Autodesk Inventor part; units mm, degrees
ref_plane "YZ Plane" through (0, 0, 0) normal (1, 0, 0) x (0, 1, 0)
ref_plane "XZ Plane" through (0, 0, 0) normal (0, 1, 0) x (-1, 0, 0)
ref_plane "XY Plane" through (0, 0, 0) normal (0, 0, 1) x (1, 0, 0)
sketch "Sketch1" plane through (0, 0, 0) normal (0, 1, 0) x (-1, 0, 0)
  line L0 (56, 0) -> (-56, 0)
  line L1 (0, -156) -> (0, 26)
  line L2 (40, 0) -> (-40, 0)
  line L3 (-40, 0) -> (-40, -130)
  line L4 (-40, -130) -> (40, -130)
  line L5 (40, -130) -> (40, 0)
  point P0 (0, 0)
  point P1 (0, 0)
  dimension "d0" = 80
  dimension "d1" = 130
  dimension "d2" = 40
extrude "Extrusion1" add sketch "Sketch1" along normal blind 60
sketch "Sketch2" plane through (0, 60, 0) normal (0, 1, 0) x (1, 0, 0)
  line L0 (-35, 5) -> (35, 5)
  line L1 (35, 5) -> (35, 125)
  line L2 (35, 125) -> (-35, 125)
  line L3 (-35, 125) -> (-35, 5)
  line L4 (-40, 130) -> (-40, 0)
  line L5 (-40, 0) -> (40, 0)
  point P0 (0, 0)
  dimension "d5" = 70
  dimension "d6" = 120
  dimension "d7" = 5
  dimension "d8" = 5
extrude "Extrusion2" cut sketch "Sketch2" against normal blind 50
sketch "Sketch3" plane through (40, 0, 0) normal (1, 0, 0) x (0, 0, -1)
  line L0 (113, 48) -> (123, 48)
  line L1 (123, 48) -> (123, 30)
  line L2 (123, 30) -> (113, 30)
  line L3 (113, 30) -> (113, 48)
  line L4 (130, 0) -> (130, 60)
  line L5 (0, 60) -> (130, 60)
  line L6 (98, 48) -> (108, 48)
  line L7 (108, 48) -> (108, 30)
  line L8 (108, 30) -> (98, 30)
  line L9 (98, 30) -> (98, 48)
  point P0 (0, 0)
  dimension "d11" = 10
  dimension "d12" = 18
  dimension "d13" = 7
  dimension "d14" = 12
  dimension "d15" = 10
  dimension "d16" = 18
  dimension "d17" = 5
extrude "Extrusion3" cut sketch "Sketch3" against normal blind 5
sketch "Sketch4" plane through (40, 0, 0) normal (1, 0, 0) x (0, 0, -1)
  circle A0 centre (115, 15) radius 5
  line L0 (0, 0) -> (130, 0)
  line L1 (130, 0) -> (130, 60)
  dimension "d20" = 10
  dimension "d21" = 15
  dimension "d22" = 15
extrude "Extrusion4" cut sketch "Sketch4" against normal blind 5
sketch "Sketch6" plane through (0, 10, 0) normal (0, 1, 0) x (1, 0, 0)
  line L0 (-35, 125) -> (35, 125)
  line L1 (-35, 5) -> (-35, 125)
  line L2 (35, 5) -> (-35, 5)
  line L3 (35, 115) -> (35, 5)
  line L4 (35, 125) -> (35, 115)
  line L5 (-35, 88) -> (30, 88)
  line L6 (30, 88) -> (30, 78)
  line L7 (30, 78) -> (-35, 78)
  line L8 (-35, 78) -> (-35, 88)
  line L9 (25, 125) -> (25, 88)
  line L10 (25, 88) -> (30, 88)
  line L11 (30, 88) -> (30, 125)
  point P0 (0, 0)
  dimension "d30" = 65
  dimension "d31" = 10
extrude "Extrusion6" add sketch "Sketch6" along normal blind 25 contours L5 L6 L7 L1
sketch "Sketch7" plane through (0, 10, 0) normal (0, 1, 0) x (1, 0, 0)
  line L0 (30, 78) -> (-35, 78)
  line L1 (-35, 5) -> (-35, 78)
  line L2 (35, 5) -> (-35, 5)
  line L3 (35, 115) -> (35, 5)
  line L4 (35, 125) -> (35, 115)
  line L5 (-35, 125) -> (35, 125)
  line L6 (30, 88) -> (30, 78)
  line L7 (-35, 57) -> (30, 57)
  line L8 (30, 57) -> (30, 47)
  line L9 (30, 47) -> (-35, 47)
  line L10 (-35, 47) -> (-35, 57)
  line L11 (30, 88) -> (30, 125)
  line L12 (-35, 88) -> (30, 88)
  line L13 (-35, 88) -> (-35, 125)
  point P0 (0, 0)
  dimension "d34" = 65
  dimension "d35" = 10
  dimension "d36" = 21
extrude "Extrusion7" add sketch "Sketch7" along normal blind 25 contours L7 L8 L9 L1
sketch "Sketch8" plane through (0, 10, 0) normal (0, 1, 0) x (1, 0, 0)
  line L0 (-35, 57) -> (30, 57)
  line L1 (30, 57) -> (30, 47)
  line L2 (30, 47) -> (-35, 47)
  line L3 (-35, 5) -> (-35, 47)
  line L4 (35, 5) -> (-35, 5)
  line L5 (35, 115) -> (35, 5)
  line L6 (35, 125) -> (35, 115)
  line L7 (-35, 125) -> (35, 125)
  line L8 (30, 88) -> (30, 78)
  line L9 (30, 78) -> (-35, 78)
  line L10 (-35, 57) -> (-35, 78)
  line L11 (-35, 78) -> (-25, 78)
  line L12 (-25, 78) -> (-25, 57)
  line L13 (-25, 57) -> (-35, 57)
  line L14 (-35, 57) -> (-35, 78)
  line L15 (16, 58) -> (16, 79)
  line L16 (16, 79) -> (26, 79)
  line L17 (26, 79) -> (26, 57)
  line L18 (26, 57) -> (16, 57)
  line L19 (16, 57) -> (16, 79)
  line L20 (30, 57) -> (-35, 57)
  line L21 (-35, 88) -> (-35, 125)
  line L22 (-35, 88) -> (30, 88)
  point P0 (0, 0)
  dimension "d39" = 10
  dimension "d40" = 10
  dimension "d41" = 41
extrude "Extrusion8" add sketch "Sketch8" along normal blind 20 contours L10 L9 L12 L0 | L19 L15 L9 L17 L0 | L15 L16 L17 L9
sketch "Sketch10" plane through (-40, 0, 0) normal (0, 0, 1) x (1, 0, 0)
  circle A0 centre (22, 40) radius 1.625
  circle A1 centre (40, 40) radius 1.625
  circle A2 centre (58, 40) radius 1.625
  line L0 (0, 0) -> (0, 60)
  line L1 (0, 0) -> (80, 0)
  line L2 (80, 0) -> (80, 60)
  line L3 (0, 60) -> (80, 60)
  line L4 (0, 0) -> (0, 60)
  point P0 (40, 0)
  dimension "d49" = 3.25
  dimension "d51" = 3.25
  dimension "d53" = 3.25
  dimension "d55" = 18
  dimension "d56" = 18
  dimension "d59" = 22
  dimension "d60" = 22
  dimension "d61" = 20
extrude "Extrusion10" cut sketch "Sketch10" against normal blind 10 contours A0 | A1 | A2
sketch "Sketch11" plane through (-40, 0, 0) normal (0, 0, 1) x (1, 0, 0)
  circle A0 centre (13, 35) radius 0.75
  circle A1 centre (31, 35) radius 0.75
  circle A2 centre (49, 35) radius 0.75
  circle A3 centre (67, 35) radius 0.75
  circle A4 centre (40, 40) radius 1.625
  circle A5 centre (22, 40) radius 1.625
  circle A6 centre (58, 40) radius 1.625
  line L0 (0, 0) -> (80, 0)
  line L1 (80, 0) -> (80, 60)
  line L2 (0, 60) -> (80, 60)
  line L3 (0, 0) -> (0, 60)
  dimension "d64" = 1.5
  dimension "d65" = 1.5
  dimension "d66" = 1.5
  dimension "d67" = 1.5
  dimension "d71" = 18
  dimension "d73" = 18
  dimension "d75" = 18
  dimension "d76" = 13
  dimension "d77" = 13
  dimension "d78" = 5
  dimension "d79" = 5
extrude "Extrusion11" cut sketch "Sketch11" against normal blind 10 contours A0 | A1 | A2 | A3
sketch "Sketch12" plane through (0, 60, 0) normal (0, 1, 0) x (1, 0, 0)
  line L0 (-44.75, 134.75) -> (44.75, 134.75)
  line L1 (44.75, 134.75) -> (44.75, -4.75)
  line L2 (44.75, -4.75) -> (-44.75, -4.75)
  line L3 (-44.75, -4.75) -> (-44.75, 134.75)
  line L4 (35, 125) -> (35, 5)
  line L5 (35, 5) -> (-35, 5)
  line L6 (-35, 5) -> (-35, 125)
  line L7 (-35, 125) -> (35, 125)
  line L8 (-40, 0) -> (40, 0)
  line L9 (40, 0) -> (40, 130)
  line L10 (40, 130) -> (-40, 130)
  line L11 (-40, 130) -> (-40, 0)
  line L12 (-40, 130) -> (-40, 0)
  line L13 (-40, 130) -> (40, 130)
  line L14 (40, 130) -> (40, 0)
  line L15 (40, 0) -> (-40, 0)
  line L16 (-40, 0) -> (-40, 130)
  point P0 (0, 0)
  dimension "d82" = 4.75
  dimension "d83" = 4.75
  dimension "d84" = 4.75
  dimension "d85" = 4.75
extrude "Extrusion12" add sketch "Sketch12" against normal blind 5 contours L0 L1 L2 L3
sketch "Sketch15" plane through (0, 55, 0) normal (0, -1, 0) x (1, 0, 0)
  line L0 (40, 0) -> (-40, 0)
  line L1 (40, -130) -> (40, 0)
  line L2 (-40, -130) -> (40, -130)
  line L3 (-40, 0) -> (-40, -130)
  line L4 (-44.75, -134.75) -> (44.75, -134.75)
  line L5 (44.75, -134.75) -> (44.75, 4.75)
  line L6 (44.75, 4.75) -> (-44.75, 4.75)
  line L7 (-44.75, 4.75) -> (-44.75, -134.75)
  line L8 (-40, 0) -> (40, 0)
  line L9 (-40, -130) -> (-40, 0)
  line L10 (40, -130) -> (-40, -130)
  line L11 (40, 0) -> (40, -130)
  circle A0 centre (-42.375, 2.375) radius 1.625
  circle A1 centre (42.375, 2.375) radius 1.625
  circle A2 centre (42.375, -132.375) radius 1.625
  circle A3 centre (-42.375, -132.375) radius 1.625
  point P0 (0, 0)
  dimension "d91" = 3.25
  dimension "d92" = 2.375
  dimension "d93" = 2.375
  dimension "d94" = 3.25
  dimension "d95" = 2.375
  dimension "d96" = 2.375
  dimension "d97" = 3.25
  dimension "d98" = 2.375
  dimension "d99" = 2.375
  dimension "d100" = 3.25
  dimension "d101" = 2.375
  dimension "d102" = 2.375
extrude "Extrusion13" cut sketch "Sketch15" against normal blind 5 contours A0 | A1 | A2 | A3
sketch "Sketch16" plane through (0, 30, 0) normal (0, 1, 0) x (1, 0, 0)
  line L0 (16, 78) -> (26, 78)
  line L1 (16, 78) -> (16, 57)
  line L2 (26, 57) -> (16, 57)
  line L3 (26, 57) -> (26, 78)
  line L4 (16, 57) -> (16, 78)
  line L5 (26, 78) -> (26, 57)
  line L6 (16, 74.5) -> (26, 74.5)
  line L7 (26, 74.5) -> (26, 60.5)
  line L8 (26, 60.5) -> (16, 60.5)
  line L9 (16, 60.5) -> (16, 74.5)
  point P0 (0, 0)
  dimension "d105" = 3.5
  dimension "d106" = 3.5
extrude "Extrusion14" cut sketch "Sketch16" against normal blind 20 contours L6 L3 L8 L1
properties part number "mien_arm"
Work out the finished part from the listing and answer in its coordinate system (mm). A direction names the side the tool comes from. Coordinates: 2 decimals unless noted, no trailing zeros. Loops run counter-clockwise (first coordinate to the right, second up) from the corner with the lowest first, then second, coordinate; pieces in that order, holes last. Notation, with made-up numbers: (-17.75, -15.75) -> (36.25, -15.75) arc R11 ccw to (36.25, -11.75) -> close; hole circle Ø4 at (55.5, 77.25). An arc over 180 degrees is marked (long way). Answer as CSV lines item,"result".
1) Straight lines are drawn through the part: probe 1 along Y at (x, z) = (36, -115); probe 2 along Z at (x, y) = (-9.5, 29); probe 3 along Z at (x, y) = (18.5, 26.5). For each, find the intervals that lie inside material, in ascending order.
A:
probe 1,"y = 0 to 10, 20 to 30, 48 to 60"
probe 2,"z = -130 to -125, -88 to -78, -57 to -47, -5 to 0"
probe 3,"z = -130 to -125, -88 to -74.5, -60.5 to -47, -5 to 0"
2) The part is cut by section C-C (z = -27). Give the vertices of the cut face in (x, y), and give its area (3 significant figures).
A:
outline,"(-44.75, 55) -> (-40, 55) -> (-40, 0) -> (40, 0) -> (40, 55) -> (44.75, 55) -> (44.75, 60) -> (35, 60) -> (35, 10) -> (-35, 10) -> (-35, 60) -> (-44.75, 60) -> close"
area,"1,350 mm²"
3) The part is cut by section A-A (y = 40). Give the vertices of the cut face in (x, z) (3 decimals).
A:
outline,"(-40, -130) -> (40, -130) -> (40, -123) -> (35, -123) -> (35, -125) -> (-35, -125) -> (-35, -5) -> (-19.625, -5) -> (-19.625, 0) -> (-40, 0) -> close; (-16.375, -5) -> (-1.625, -5) -> (-1.625, 0) -> (-16.375, 0) -> close; (1.625, -5) -> (16.375, -5) -> (16.375, 0) -> (1.625, 0) -> close; (19.625, -5) -> (35, -5) -> (35, -98) -> (40, -98) -> (40, 0) -> (19.625, 0) -> close; (35, -113) -> (40, -113) -> (40, -108) -> (35, -108) -> close"
4) The part is cut by section D-D (x = 12.5). Give the vertices of the cut face in (y, z).
A:
outline,"(0, -130) -> (55, -130) -> (55, -134.75) -> (60, -134.75) -> (60, -125) -> (10, -125) -> (10, -88) -> (35, -88) -> (35, -78) -> (10, -78) -> (10, -57) -> (35, -57) -> (35, -47) -> (10, -47) -> (10, -5) -> (60, -5) -> (60, 4.75) -> (55, 4.75) -> (55, 0) -> (0, 0) -> close"
5) The part is cut by section B-B (x = 0). Give the vertices of the cut face in (y, z) (3 decimals), and give its area (3 significant figures).
A:
outline,"(0, -130) -> (55, -130) -> (55, -134.75) -> (60, -134.75) -> (60, -125) -> (10, -125) -> (10, -88) -> (35, -88) -> (35, -78) -> (10, -78) -> (10, -57) -> (35, -57) -> (35, -47) -> (10, -47) -> (10, -5) -> (38.375, -5) -> (38.375, 0) -> (0, 0) -> close; (41.625, -5) -> (60, -5) -> (60, 4.75) -> (55, 4.75) -> (55, 0) -> (41.625, 0) -> close"
area,"2,330 mm²"
6) For faces 4 (the face through (37.535, 13.085, -119.619)), 5 (the face through (-2, 22, -47)), 6 (the face through (-1, 27, 0)), determine the directions among +Z, -Z, +X, -X, +Y, -Y from which every point of the face is accessible in a straight line to the end or side of a thin tool.
A:
face 4,"+X"
face 5,"+Y"
face 6,"+Z, +X, -X, -Y"
7) For a pull along X with two mould halves and no side action, classify faces 1 (the face through (38, 30, -103)), 2 (the face through (0, 35, -125)), 3 (the face through (-44.75, 58, -64)) as released by +X, released by -X, zero draft, split by the parting line, or undercut.
A:
face 1,"zero draft"
face 2,"undercut"
face 3,"released by -X"
8) Flat-ended cylindrical pins translate along their axes: pin 1 (1.8 mm diameter, centred on y = 18.5, z = -76.5, fed in from -X); pin 2 (1.4 mm diameter, centred on x = 9, y = 35, fed in from +Z); pin 3 (2.5 mm diameter, centred on x = -18, y = 40, fed in from +Z). Find the tip coordinate at first contact, or state that the pin passes through.
A:
pin 1,"stops at x = -40"
pin 2,"stops at z = -47"
pin 3,"stops at z = -125"
